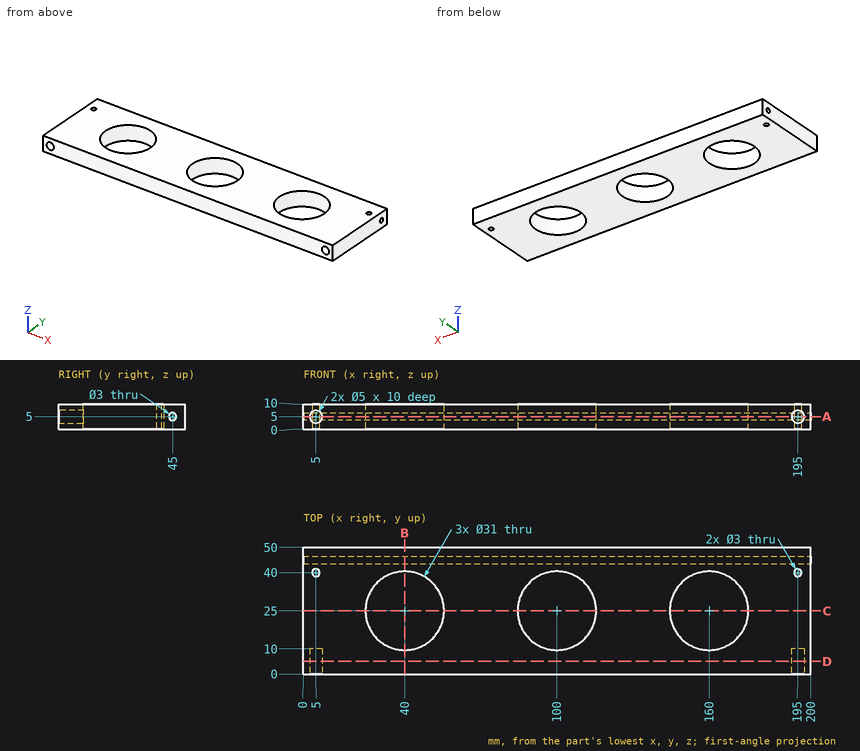
Geometry check sheet. Reference: drawing and pictorial views, mm from the part's lowest x, y, z. Coordinates: 2 decimals unless noted, no trailing zeros. Loops run counter-clockwise (first coordinate to the right, second up) from the corner with the lowest first, then second, coordinate; pieces in that order, holes last. Notation, with made-up numbers: M 40.5,-20.75 L 82.5,-20.75 A23 cw 82.5,9.25 Z; hole C 48,8.25 d2. An arc over 180 degrees is marked long. One line per item, written item: value.
1. Section check A-A on z = 5. Record the cut outline in (x, y), plus the area to 3 significant figures.
Answers follow:
outline: M 0,0 L 2.5,0 L 2.5,10 L 7.5,10 L 7.5,0 L 192.5,0 L 192.5,10 L 197.5,10 L 197.5,0 L 200,0 L 200,43.5 L 0,43.5 Z; M 0,46.5 L 200,46.5 L 200,50 L 0,50 Z; hole C 5,40 d3; hole C 40,25 d31; hole C 100,25 d31; hole C 160,25 d31; hole C 195,40 d3
area: 7,020 mm^2
2. Section check C-C on y = 25. Record the cut outline in (x, z).
Answers follow:
outline: M 0,0 L 24.5,0 L 24.5,10 L 0,10 Z; M 55.5,0 L 84.5,0 L 84.5,10 L 55.5,10 Z; M 115.5,0 L 144.5,0 L 144.5,10 L 115.5,10 Z; M 175.5,0 L 200,0 L 200,10 L 175.5,10 Z
3. Section check D-D on y = 5. Record the cut outline in (x, z), plus the area to 3 significant figures.
Answers follow:
outline: M 0,0 L 200,0 L 200,10 L 0,10 Z; hole C 5,5 d5; hole C 195,5 d5
area: 1,960 mm^2
4. Gauge pin test, flat end, axial feed: P1, Ø4, axis at x = 195, z = 5, coming from the -Y side. Record the tip position at first contact, or that the pin passes through.
Answers follow:
P1: y = 10
5. Section check B-B on x = 40. Record the cut outline in (y, z).
Answers follow:
outline: M 0,0 L 9.5,0 L 9.5,10 L 0,10 Z; M 40.5,0 L 50,0 L 50,10 L 40.5,10 Z; hole C 45,5 d3
6. Material ranges on line 1 along X through (y, z) = (24.5, 6.75); line 2 along Y through (x, z) = (160.5, 2.5); line 3 along X through (y, z) = (17, 2), recorded low to high. Write a range as from..to.
Answers follow:
line 1: 0..24.51, 55.49..84.51, 115.49..144.51, 175.49..200
line 2: 0..9.51, 40.49..50
line 3: 0..26.72, 53.28..86.72, 113.28..146.72, 173.28..200
